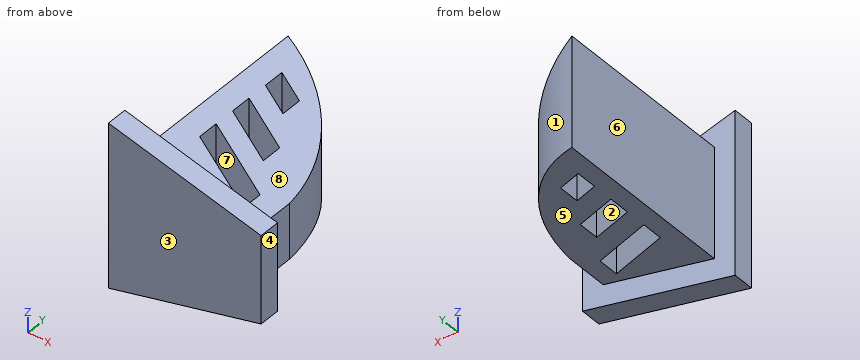
from build123d import *

# Parameters (mm, degrees)
EXTRUDE1_DEPTH = 15
EXTRUDE2_DEPTH = 130
EXTRUDE3_DEPTH = 65


with BuildPart() as part:
    # Sketch1 → Extrude1 (new body)
    with BuildSketch(Plane(origin=(0, 0, 0), x_dir=(1, 0, 0), z_dir=(0, 1, 0))):
        Polygon((15, -11.711646096), (-95, -39.211646096), (-95, 79.211646096), (15, 51.711646096), align=None)
    extrude(amount=EXTRUDE1_DEPTH)

    # Sketch2 → Extrude2 (add)
    with BuildSketch(Plane(origin=(0, 15, 0), x_dir=(1, 0, 0), z_dir=(0, 1, 0))):
        Polygon((0, 0), (0, 40), (-80, 60), (-80, -20), align=None)
    extrude(amount=EXTRUDE2_DEPTH)

    # Sketch3 → Extrude3 (cut, symmetric)
    with BuildSketch(Plane.XY):
        with BuildLine():
            Line((-80, 145), (0, 145))
            Line((0, 145), (0, 45))
            ThreePointArc((0, 45), (-25.545271603, 106.563782718), (-80, 145))
        make_face()
        Polygon((-65, 120.30999778), (-65, 105.30999778), (-45, 95.983844617), (-45, 110.983844617), align=None)
        Polygon((-65, 45.30999778), (-15, 21.994614872), (-15, 36.994614872), (-65, 60.30999778), align=None)
        Polygon((-65, 75.30999778), (-30, 58.989229745), (-30, 73.989229745), (-65, 90.30999778), align=None)
    extrude(amount=EXTRUDE3_DEPTH, both=True, mode=Mode.SUBTRACT)


solid = part.part
Verification items for the finished model (mm, model axes). Face numbers are marked on the shaded views. A direction names the side the tool comes from. Round coordinates to 2 decimals unless told otherwise and drop trailing zeros. Order: outer loops, then holes, each group sorted by start corner. A loop starts at its lowest first (then second) coordinate and runs counter-clockwise, first axis right, second up. Notation, with made-up numbers: (9, -18.75) -> (66, -18.75) arc R27 ccw to (66, 5.25) -> close; hole circle Ø3 at (29, -5). An arc over 180 degrees is marked (long way). Put each result on its own line as item: value.
1) Section check C-C (y = 69.5). Record the cut outline in (x, z).
Final values:
outline: (-80, -60) -> (-52.54, -53.14) -> (-52.54, 13.14) -> (-80, 20) -> close; (-30, -47.5) -> (-5.39, -41.35) -> (-5.39, 1.35) -> (-30, 7.5) -> close
2) Depth check by flat-ended pin: pin 1 (1.5 mm diameter, centred on x = -39.5, z = -51.5, fed in from +Y); pin 2 (1.5 mm diameter, centred on x = -50.5, z = -31, fed in from +Y); pin 3 (9 mm diameter, centred on y = 26, z = -12, fed in from +X). Enter the tip coordinate at first touch or a pass-through.
Final values:
pin 1: stops at y = 15
pin 2: stops at y = 130.47
pin 3: stops at x = 0
3) Set-up check for the marked faces 5, 6, 7 and 8: record each of +Z, -Z, +X, -X, +Y, -Y from which the full face is reachable in a straight line by a thin tool's end or side.
Final values:
face 5: -Z, +X, +Y
face 6: +Z, -Z, -X, +Y
face 7: +Z, -Z
face 8: +Z, +X, +Y
4) Material ranges on line 1 (Y direction, x = -57.5, z = 2.5); line 2 (Y direction, x = -51, z = -42); line 3 (Y direction, x = -47.5, z = 13), recorded low to high.
Final values:
line 1: y = 0 to 41.81, 56.81 to 71.81, 86.81 to 101.81, 116.81 to 134.49
line 2: y = 0 to 38.78, 53.78 to 68.78, 83.78 to 98.78, 113.78 to 130.3
line 3: y = 0 to 15
5) Section check A-A (z = -11.5). Record the cut outline in (x, y), then the cut area to 3 significant figures.
Final values:
outline: (-95, 0) -> (15, 0) -> (15, 15) -> (0, 15) -> (0, 45) arc R120 ccw to (-80, 145) -> (-80, 15) -> (-95, 15) -> close; hole (-65, 45.31) -> (-15, 21.99) -> (-15, 36.99) -> (-65, 60.31) -> close; hole (-65, 75.31) -> (-30, 58.99) -> (-30, 73.99) -> (-65, 90.31) -> close; hole (-65, 105.31) -> (-45, 95.98) -> (-45, 110.98) -> (-65, 120.31) -> close
area: 8,080 mm^2
6) Mould release check, pull along Y, two halves, no side actions. Record for the marked faces 1, 2, 3 and 4: +Y half, -Y half, draft (parallel to the pull), parting line (faces both ways), or undercut.
Final values:
face 1: +Y half
face 2: undercut
face 3: -Y half
face 4: draft
7) Section check B-B (x = -26.5). Record the cut outline in (y, z) (3 decimals).
Final values:
outline: (0, -62.087) -> (15, -62.087) -> (15, -46.625) -> (27.357, -46.625) -> (27.357, 6.625) -> (15, 6.625) -> (15, 22.087) -> (0, 22.087) -> close; (42.357, -46.625) -> (107.742, -46.625) -> (107.742, 6.625) -> (42.357, 6.625) -> close
8) Section check D-D (x = -51.5). Record the cut outline in (y, z) (3 decimals), then the cut area to 3 significant figures.
Final values:
outline: (0, -68.337) -> (15, -68.337) -> (15, -52.875) -> (39.015, -52.875) -> (39.015, 12.875) -> (15, 12.875) -> (15, 28.337) -> (0, 28.337) -> close; (54.015, -52.875) -> (69.015, -52.875) -> (69.015, 12.875) -> (54.015, 12.875) -> close; (84.015, -52.875) -> (99.015, -52.875) -> (99.015, 12.875) -> (84.015, 12.875) -> close; (114.015, -52.875) -> (130.646, -52.875) -> (130.646, 12.875) -> (114.015, 12.875) -> close
area: 6,100 mm^2
